from build123d import *

# Parameters (mm, degrees)
SKETCH1_W                                          = 234.95
SKETCH1_H                                          = 203.2
BOSS_EXTRUDE1_DEPTH                                = 6.35
SKETCH2_R                                          = 14.2748
CUT_EXTRUDE1_DEPTH                                 = 7.35
CSK_FOR_10_FLAT_HEAD_MACHINE_SCREW_100_D           = 5.6134
CSK_FOR_10_FLAT_HEAD_MACHINE_SCREW_100_CSINK_D     = 17.78
CSK_FOR_10_FLAT_HEAD_MACHINE_SCREW_100_CSINK_ANGLE = 90
CSK_FOR_10_FLAT_HEAD_MACHINE_SCREW_2_D             = 5.6134
CSK_FOR_10_FLAT_HEAD_MACHINE_SCREW_2_CSINK_D       = 17.78
CSK_FOR_10_FLAT_HEAD_MACHINE_SCREW_2_CSINK_ANGLE   = 90


with BuildPart() as part:
    # Sketch1 → Boss-Extrude1 (new body)
    with BuildSketch(Plane.XY):
        Rectangle(SKETCH1_W, SKETCH1_H)
    extrude(amount=BOSS_EXTRUDE1_DEPTH)

    # Sketch2 → Cut-Extrude1 (cut, through all)
    with BuildSketch(Plane.XY.offset(6.35)):
        with Locations((61.595, 74.93)):
            Circle(SKETCH2_R)
    extrude(amount=-CUT_EXTRUDE1_DEPTH, mode=Mode.SUBTRACT)

    # CSK for _10 Flat Head Machine Screw _100 (through all)
    with Locations(Plane(origin=(271.17770657, -265.595089466, -36.034392524), x_dir=(-0.990861087, 0, 0.134886274), z_dir=(0.134886274, 0, 0.990861087))):
        with Locations((333.441972913, -227.495089466), (333.441972913, -252.895089466), (333.441972913, -329.095089466), (333.441972913, -354.495089466)):
            CounterSinkHole(CSK_FOR_10_FLAT_HEAD_MACHINE_SCREW_100_D / 2, CSK_FOR_10_FLAT_HEAD_MACHINE_SCREW_100_CSINK_D / 2, counter_sink_angle=CSK_FOR_10_FLAT_HEAD_MACHINE_SCREW_100_CSINK_ANGLE)

    # CSK for _10 Flat Head Machine Screw  2 (through all)
    with Locations(Plane(origin=(271.520317707, -265.595089466, -33.517605364), x_dir=(-0.990861087, 0, 0.134886274), z_dir=(0.134886274, 0, 0.990861087))):
        with Locations((308.041972913, -252.895089466), (308.041972913, -227.495089466), (308.041972913, -329.095089466), (308.041972913, -354.495089466)):
            CounterSinkHole(CSK_FOR_10_FLAT_HEAD_MACHINE_SCREW_2_D / 2, CSK_FOR_10_FLAT_HEAD_MACHINE_SCREW_2_CSINK_D / 2, counter_sink_angle=CSK_FOR_10_FLAT_HEAD_MACHINE_SCREW_2_CSINK_ANGLE)


solid = part.part
Geometry: final body of the model. Coordinates: model frame, mm. Give positions to 0.01 mm unless a question says otherwise; leave off trailing zeros. Write each loop counter-clockwise with the first axis right and the second up, starting at its lowest first coordinate (ties: lowest second). Pieces come first, ordered by that corner, then holes. Notation, with made-up numbers: (75, 87) - (108, 87) arc R14 ccw to (108, 94) - close; hole circle Ø7 at (4.25, 18.25). An arc over 180 degrees is marked (long way). Return JSON: item names as keys, results as strings. Group by question number.
1) Mould query, pull axis X, two halves, no side actions, for faces 1 (the conical face through (-31.677, -36.922, 1.888)), 2 (the flat face through (-2, 1, 6.35)), 3 (the flat face through (-117.475, -1, 3)). Classes: released by +X, released by -X, zero draft, split by the parting line, or undercut.
2) Section B-B on z = 5. State how many separate pieces and enclosed holes the cut face has, plus the area to 3 significant figures.
3) First-contact query: P1, Ø5, axis at x = -43.5, y = 71, coming from the -Z side. Flat tip, straight axial feed; report the tip coordinate or a pass-through.
4) Line query: line 1 (Y direction, x = 67, z = 5.75); line 2 (Y direction, x = 53.5, z = 4); line 3 (Z direction, x = -64, y = 66). Output: solid intervals per line, ascending.
5) Section A-A on y = 74.93. Return the cut outline in (x, z) (3 decimals).
Filled in:
{
 "1": {"face 1": "undercut", "face 2": "zero draft", "face 3": "released by -X"},
 "2": {"separate pieces": "1", "enclosed holes": "9", "area": "46,300 mm^2"},
 "3": {"P1": "stops at z = 0"},
 "4": {"line 1": "y = -101.6 to 61.72, 88.14 to 101.6", "line 2": "y = -101.6 to 63.17, 86.69 to 101.6", "line 3": "z = 0 to 5.64"},
 "5": {"outline": "(-117.475, 0) - (47.32, 0) - (47.32, 6.35) - (-117.475, 6.35) - close; (75.87, 0) - (117.475, 0) - (117.475, 6.35) - (75.87, 6.35) - close"}
}
